from build123d import *

# Parameters (mm, degrees)
CROQUIS1_R              = 15.575
CROQUIS1_R_2            = 13.075
SALIENTE_EXTRUIR1_DEPTH = 4
SALIENTE_EXTRUIR2_DEPTH = 4
SALIENTE_EXTRUIR3_DEPTH = 2.45
CROQUIS4_R              = 1.625
CORTAR_EXTRUIR1_DEPTH   = 19.025


with BuildPart() as part:
    # Croquis1 → Saliente-Extruir1 (new body)
    with BuildSketch(Plane(origin=(0, 0, 0), x_dir=(1, 0, 0), z_dir=(0, 1, 0))):
        Circle(CROQUIS1_R)
        Circle(CROQUIS1_R_2, mode=Mode.SUBTRACT)
    extrude(amount=SALIENTE_EXTRUIR1_DEPTH)

    # Croquis2 → Saliente-Extruir2 (add)
    with BuildSketch(Plane(origin=(0, 0, 0), x_dir=(1, 0, 0), z_dir=(0, 1, 0))):
        with BuildLine():
            Line((20.575, 2.45), (10.410630983, 11.584445932))
            ThreePointArc((10.410630983, 11.584445932), (15.575, 0), (10.410630983, -11.584445932))
            Line((10.410630983, -11.584445932), (20.575, -2.45))
            Line((20.575, -2.45), (20.575, 2.45))
        make_face()
    extrude(amount=SALIENTE_EXTRUIR2_DEPTH)

    # Croquis3 → Saliente-Extruir3 (add, symmetric)
    with BuildSketch(Plane.XY):
        with BuildLine():
            Line((20.575, 4), (20.575, 0))
            Line((20.575, 0), (20.992424305, 0))
            ThreePointArc((20.992424305, 0), (30.575, 2), (20.992424305, 4))
            Line((20.992424305, 4), (20.575, 4))
        make_face()
    extrude(amount=SALIENTE_EXTRUIR3_DEPTH, both=True)

    # Croquis4 → Cortar-Extruir1 (cut, through all)
    with BuildSketch(Plane.XY.offset(2.45)):
        with Locations((25.575, 2)):
            Circle(CROQUIS4_R)
    extrude(amount=-CORTAR_EXTRUIR1_DEPTH, mode=Mode.SUBTRACT)


solid = part.part
Design review of the part built by this model. Coordinates are the model's own, in mm. A direction names the side the tool comes from. Give positions to 0.01 mm unless a question says otherwise; leave off trailing zeros. Loops run counter-clockwise (first coordinate to the right, second up) from the corner with the lowest first, then second, coordinate; pieces in that order, holes last. Notation, with made-up numbers: M 34,72.25 L 44,72.25 A18 ccw 44,82.25 Z; hole C 45,12.25 d10. An arc over 180 degrees is marked long. Write item = value, one per line.
Q1. We need section C-C (z = 0). Give the boundary of the cut face in (x, y) (3 decimals), plus the area to 3 significant figures.
Output values:
outline = M -15.575,0 L -13.075,0 L -13.075,4 L -15.575,4 Z; M 13.075,0 L 20.992,0 A5 ccw long 20.992,4 L 13.075,4 Z; hole C 25.575,2 d3.25
area = 111 mm^2
Q2. For faces 4 (the flat face through (13.5, 0, 0.1)), 5 (the flat face through (24, 3, 2.45)), 6 (the flat face through (24, 3, -2.45)), list the 3-axis set-ups (+Z, -Z, +X, -X, +Y, -Y) from which the entire face can be reached by the end or side of a thin tool; tool diameter is ignored.
Output values:
face_4 = +Z, -Z, -X, -Y
face_5 = +Z, +X, +Y, -Y
face_6 = -Z, +X, +Y, -Y
Q3. We need section A-A (y = 2). Give the boundary of the cut face in (x, z) (3 decimals), plus the area to 3 significant figures.
Output values:
outline = M 10.411,-11.584 L 20.575,-2.45 L 23.95,-2.45 L 23.95,2.45 L 20.575,2.45 L 10.411,11.584 A15.575 ccw long Z; M 27.2,-2.45 L 30.575,-2.45 L 30.575,2.45 L 27.2,2.45 Z; hole C 0,0 d26.15
area = 318 mm^2
Q4. We need section D-D (z = 4.5). Give the boundary of the cut face in (x, y).
Output values:
outline = M -14.91,0 L -12.28,0 L -12.28,4 L -14.91,4 Z; M 12.28,0 L 18.29,0 L 18.29,4 L 12.28,4 Z
Q5. Draft analysis for pull direction Y (two halves, no side actions). For faces 1 (the cylindrical face through (-2.834, 1.972, 12.764)), 2 (the flat face through (12, 4, 6)), 3 (the cylindrical face through (25.36, 3.61, 0.03)), state which applies: +Y half, -Y half, draft (parallel to the pull), parting line (faces both ways), or undercut.
Output values:
face_1 = draft
face_2 = +Y half
face_3 = undercut
Q6. To check wall thickness, follow line 1 (X direction, y = 1.85, z = 0) (3 decimals); line 2 (Z direction, x = 0, y = 1.9) (3 decimals); line 3 (Y direction, x = 16, z = 0.5). State the ranges of each line that lie inside material, in increasing order. Write a range as [from, to].
Output values:
line_1 = [-15.575, -13.075], [13.075, 23.957], [27.193, 30.573]
line_2 = [-15.575, -13.075], [13.075, 15.575]
line_3 = [0, 4]
Q7. We need section B-B (x = 0). Give the boundary of the cut face in (y, z) (3 decimals).
Output values:
outline = M 0,-15.575 L 4,-15.575 L 4,-13.075 L 0,-13.075 Z; M 0,13.075 L 4,13.075 L 4,15.575 L 0,15.575 Z
Q8. Insertion check: pin 1 (10 mm diameter, centred on x = 14.5, z = -11, fed in from -Y); pin 2 (2 mm diameter, centred on y = 3, z = -2, fed in from -X); pin 3 (2 mm diameter, centred on x = 20, y = 2.5, fed in from -Z); pin 4 (15.5 mm diameter, centred on x = -2.5, z = -1, fed in from -Y). Each pin has a flat end and moves straight along its axis. Give the tip position at first contact, or say it passes through.
Output values:
pin_1 = 0
pin_2 = -15.54
pin_3 = -3.87
pin_4 = through
